Geometry check sheet. Reference: the model listing, model coordinates, mm. A direction names the side the tool comes from. Coordinates: 2 decimals unless noted, no trailing zeros. Write each loop counter-clockwise with the first axis right and the second up, starting at its lowest first coordinate (ties: lowest second). Pieces come first, ordered by that corner, then holes.
from build123d import *

# Parameters (mm, degrees)
F0_W     = 50
F0_H     = 70
F0_R     = 2.5
F0_R_2   = 2
F1_DEPTH = 6
F2_DEPTH = 2


with BuildPart() as f1:
    # F0 (on Top) → F1 (new body)
    with BuildSketch(Plane.XY):
        with Locations((25, 35)):
            Rectangle(F0_W, F0_H)
        with Locations((7, 7)):
            Circle(F0_R, mode=Mode.SUBTRACT)
        with Locations((43, 7)):
            Circle(F0_R, mode=Mode.SUBTRACT)
        Polygon((35.5, 5), (15, 5), (15, 13), (15, 53), (15, 61), (35.5, 61), (35.5, 53), (35.5, 13), align=None, mode=Mode.SUBTRACT)
        with Locations((7, 63)):
            Circle(F0_R, mode=Mode.SUBTRACT)
        with Locations((43, 63)):
            Circle(F0_R, mode=Mode.SUBTRACT)
        Polygon((15, 61), (15, 53), (24.25, 53), (24.25, 59), (26.25, 59), (26.25, 53), (35.5, 53), (35.5, 61), align=None)
        with Locations((20.25, 57)):
            Circle(F0_R_2, mode=Mode.SUBTRACT)
        with Locations((30.25, 57)):
            Circle(F0_R_2, mode=Mode.SUBTRACT)
        Polygon((15, 13), (15, 5), (35.5, 5), (35.5, 13), (26.25, 13), (26.25, 7), (24.25, 7), (24.25, 13), align=None)
        with Locations((20.25, 9)):
            Circle(F0_R_2, mode=Mode.SUBTRACT)
        with Locations((30.25, 9)):
            Circle(F0_R_2, mode=Mode.SUBTRACT)
    extrude(amount=-F1_DEPTH)

    # F0 (on Top) → F2 (cut)
    with BuildSketch(Plane.XY):
        Polygon((15, 61), (15, 53), (24.25, 53), (24.25, 59), (26.25, 59), (26.25, 53), (35.5, 53), (35.5, 61), align=None)
        with Locations((20.25, 57)):
            Circle(F0_R_2, mode=Mode.SUBTRACT)
        with Locations((30.25, 57)):
            Circle(F0_R_2, mode=Mode.SUBTRACT)
        Polygon((15, 13), (15, 5), (35.5, 5), (35.5, 13), (26.25, 13), (26.25, 7), (24.25, 7), (24.25, 13), align=None)
        with Locations((20.25, 9)):
            Circle(F0_R_2, mode=Mode.SUBTRACT)
        with Locations((30.25, 9)):
            Circle(F0_R_2, mode=Mode.SUBTRACT)
    extrude(amount=-F2_DEPTH, mode=Mode.SUBTRACT)


solid = f1.part
1. Sectioned sample at C-C, the plane y = 63. Record the boundary of the cut face in (x, z), and give its area (3 significant figures).
Computed values:
outline: (0, -6) - (4.5, -6) - (4.5, 0) - (0, 0) - close; (9.5, -6) - (40.5, -6) - (40.5, 0) - (9.5, 0) - close; (45.5, -6) - (50, -6) - (50, 0) - (45.5, 0) - close
area: 240 mm2
2. Sectioned sample at B-B, the plane y = 32. Record the boundary of the cut face in (x, z), and give its area (3 significant figures).
Computed values:
outline: (0, -6) - (15, -6) - (15, 0) - (0, 0) - close; (35.5, -6) - (50, -6) - (50, 0) - (35.5, 0) - close
area: 177 mm2
3. Gauge pin test, flat ends, axial feed: pin 1 Ø5 at (x, y) = (30.25, 9) entering from +Z; pin 2 Ø3 at (x, y) = (20.25, 57) entering from -Z. Record the tip position at first contact, or that the pin passes through.
Computed values:
pin 1: stops at z = -2
pin 2: passes through
4. Thickness scan on line 1 along Y through (x, z) = (43, -1.6); line 2 along Y through (x, z) = (30.25, -4.7); line 3 along X through (y, z) = (24, -2.15). Record the ranges inside material, lowest first.
Computed values:
line 1: y = 0 to 4.5, 9.5 to 60.5, 65.5 to 70
line 2: y = 0 to 7, 11 to 13, 53 to 55, 59 to 70
line 3: x = 0 to 15, 35.5 to 50
5. Draft check along X on faces 1 (the flat face through (50, 35, -3)), 2 (the cylindrical face through (45.31, 6.04, -2.96)), 3 (the flat face through (25, 70, -3)). Enter one of: released by +X, released by -X, zero draft, split by the parting line, or undercut.
Computed values:
face 1: released by +X
face 2: undercut
face 3: zero draft
6. Sectioned sample at A-A, the plane x = 43. Record the boundary of the cut face in (y, z), and give its area (3 significant figures).
Computed values:
outline: (0, -6) - (4.5, -6) - (4.5, 0) - (0, 0) - close; (9.5, -6) - (60.5, -6) - (60.5, 0) - (9.5, 0) - close; (65.5, -6) - (70, -6) - (70, 0) - (65.5, 0) - close
area: 360 mm2
7. Sectioned sample at D-D, the plane x = 30.25. Record the boundary of the cut face in (y, z).
Computed values:
outline: (0, -6) - (7, -6) - (7, -2) - (5, -2) - (5, 0) - (0, 0) - close; (11, -6) - (13, -6) - (13, -2) - (11, -2) - close; (53, -6) - (55, -6) - (55, -2) - (53, -2) - close; (59, -6) - (70, -6) - (70, 0) - (61, 0) - (61, -2) - (59, -2) - close
8. Access from +Z, -Z, +X, -X, +Y, -Y to the whole of each face (thin tool, end or side, straight path). Record for faces 4 (the flat face through (23, 9, -2)), 5 (the flat face through (24.25, 10, -4)), 6 (the flat face through (25, 0, -3)).
Computed values:
face 4: +Z
face 5: +Z, -Z
face 6: +Z, -Z, +X, -X, -Y
